Design review of the part shown in the three views and the two pictorial views. Dimensions are in mm from the part's minimum x, y and z. Round coordinates to 2 decimals unless told otherwise and drop trailing zeros. Order: outer loops, then holes, each group sorted by start corner. A loop starts at its lowest first (then second) coordinate and runs counter-clockwise, first axis right, second up. Notation, with made-up numbers: (-0.75, 64) -> (40.25, 64) arc R15 cw to (40.25, 71) -> close; hole circle Ø8 at (51, -22.5). An arc over 180 degrees is marked (long way). Put each result on its own line as item: value. Start each with the question number.
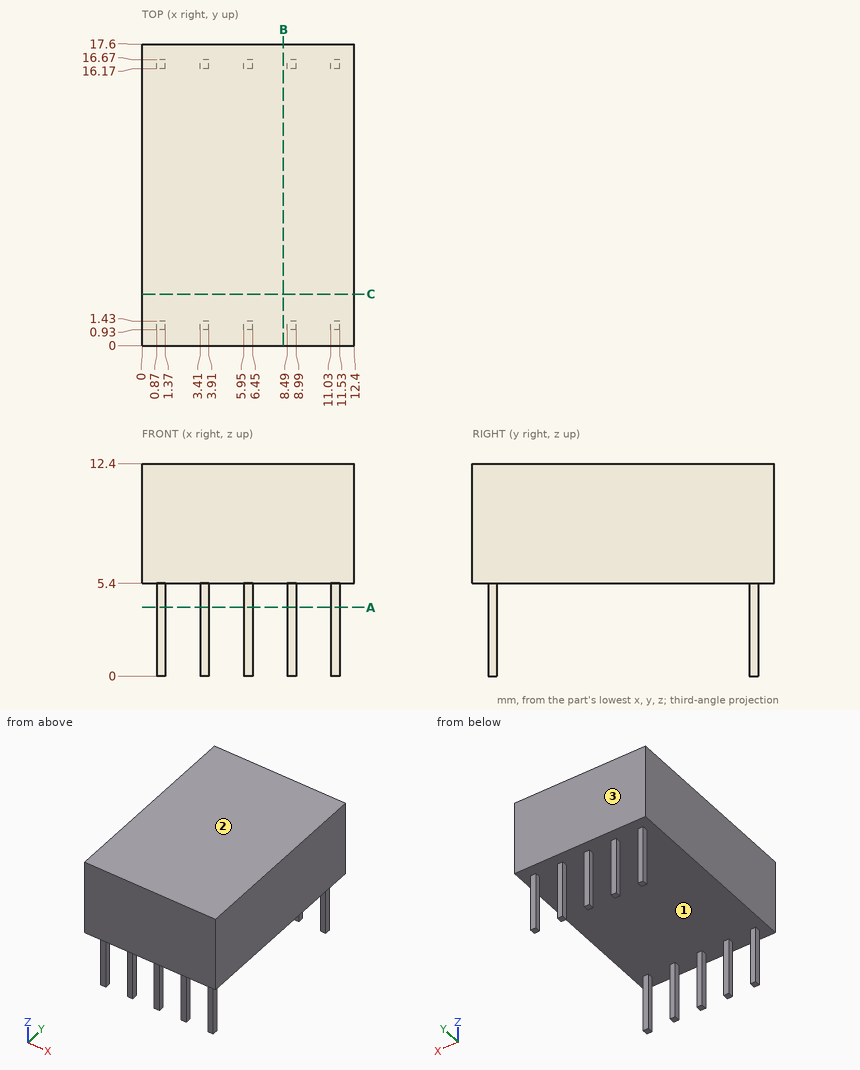
Q1. Draft analysis for pull direction Y (two halves, no side actions). For the marked faces 1, 2 and 3, state which applies: +Y half, -Y half, draft (parallel to the pull), parting line (faces both ways), or undercut.
Q2. Take a section at C-C on y = 3. Give the boundary of the cut face in (x, z).
Q3. Take a section at B-B on x = 8.25. Give the boundary of the cut face in (y, z).
Q4. Take a section at A-A on z = 4. State how many separate pieces and enclosed holes the cut face has, and give its area (3 significant figures).
Q5. Wall thickness on probe 1 along Z at (x, y) = (3, 10.5); probe 2 along Y at (x, z) = (8.75, 2.5): over which ranges is each line inside the solid? List them lowest first. Write a range as [from, to].
Q6. Clearance check with flat-ended pins moving along their axes: pin 1 Ø2 at (x, z) = (8, 7.5) entering from -Y; pin 2 Ø6 at (x, y) = (6.5, 10) entering from -Z; pin 3 Ø0.6 at (y, z) = (16.5, 2.5) entering from -X; pin 4 Ø0.6 at (x, z) = (8.5, 2) entering from +Y. State where each tip first meets the part, or that it passes through.
Calculated:
1. face 1: undercut
1. face 2: draft
1. face 3: +Y half
2. outline: (0, 5.4) -> (12.4, 5.4) -> (12.4, 12.4) -> (0, 12.4) -> close
3. outline: (0, 5.4) -> (17.6, 5.4) -> (17.6, 12.4) -> (0, 12.4) -> close
4. separate pieces: 10
4. enclosed holes: 0
4. area: 2.50 mm²
5. probe 1: z = [5.4, 12.4]
5. probe 2: y = [0.93, 1.43], [16.17, 16.67]
6. pin 1: stops at y = 0
6. pin 2: stops at z = 5.4
6. pin 3: stops at x = 0.87
6. pin 4: stops at y = 16.67
